```python
from build123d import *

# Parameters (mm, degrees)
SKETCH1_W           = 73
SKETCH1_H           = 7.175
BOSS_EXTRUDE1_DEPTH = 6
SKETCH15_W          = 4
SKETCH15_H          = 1
BOSS_EXTRUDE6_DEPTH = 1
BOSS_EXTRUDE7_START = -0.5
BOSS_EXTRUDE7_DEPTH = 7.175


with BuildPart() as part:
    # Sketch1 → Boss-Extrude1 (new body)
    with BuildSketch(Plane(origin=(0, 0, 0), x_dir=(1, 0, 0), z_dir=(0, 1, 0))):
        with Locations((0, -3.0875)):
            Rectangle(SKETCH1_W, SKETCH1_H)
    extrude(amount=BOSS_EXTRUDE1_DEPTH)

    # Sketch15 → Boss-Extrude6 (add)
    with BuildSketch(Plane(origin=(0, 6, 0), x_dir=(1, 0, 0), z_dir=(0, 1, 0))):
        with Locations((2.25, 0)):
            Rectangle(SKETCH15_W, SKETCH15_H)
        with Locations((6.75, 0)):
            Rectangle(SKETCH15_W, SKETCH15_H)
        with Locations((11.25, 0)):
            Rectangle(SKETCH15_W, SKETCH15_H)
        with Locations((15.75, 0)):
            Rectangle(SKETCH15_W, SKETCH15_H)
        with Locations((20.25, 0)):
            Rectangle(SKETCH15_W, SKETCH15_H)
        with Locations((24.75, 0)):
            Rectangle(SKETCH15_W, SKETCH15_H)
        with Locations((29.25, 0)):
            Rectangle(SKETCH15_W, SKETCH15_H)
        with Locations((33.75, 0)):
            Rectangle(SKETCH15_W, SKETCH15_H)
        with Locations((-33.75, 0)):
            Rectangle(SKETCH15_W, SKETCH15_H)
        with Locations((-29.25, 0)):
            Rectangle(SKETCH15_W, SKETCH15_H)
        with Locations((-24.75, 0)):
            Rectangle(SKETCH15_W, SKETCH15_H)
        with Locations((-20.25, 0)):
            Rectangle(SKETCH15_W, SKETCH15_H)
        with Locations((-15.75, 0)):
            Rectangle(SKETCH15_W, SKETCH15_H)
        with Locations((-11.25, 0)):
            Rectangle(SKETCH15_W, SKETCH15_H)
        with Locations((-6.75, 0)):
            Rectangle(SKETCH15_W, SKETCH15_H)
        with Locations((-2.25, 0)):
            Rectangle(SKETCH15_W, SKETCH15_H)
    extrude(amount=BOSS_EXTRUDE6_DEPTH)

    # Sketch16 → Boss-Extrude7 (add)
    with BuildSketch(Plane.XY.offset(BOSS_EXTRUDE7_START)):
        with BuildLine():
            Line((-2.54, -6), (-2.54, -9))
            Line((-2.54, -9), (-6, -9))
            Line((-6, -9), (-6, 0))
            Line((-6, 0), (6, 0))
            Line((6, 0), (6, -9))
            Line((6, -9), (2.54, -9))
            Line((2.54, -9), (2.54, -6))
            ThreePointArc((2.54, -6), (0, -3.46), (-2.54, -6))
        make_face()
    extrude(amount=BOSS_EXTRUDE7_DEPTH)


solid = part.part
```
Here's how the part is built. I have some questions about the finished solid (model axes, mm). A direction names the side the tool comes from. Give positions to 0.01 mm unless a question says otherwise; leave off trailing zeros. Loops run counter-clockwise (first coordinate to the right, second up) from the corner with the lowest first, then second, coordinate; pieces in that order, holes last. Notation, with made-up numbers: M 18,3.5 L 48,3.5 A15 ccw 48,21.5 Z; hole C 14.5,58.25 d6. An arc over 180 degrees is marked long. Put each result on its own line as item: value. Start each with the question number.
(1) Will these pins go through, and if not, where does the flat tip stop? pin 1 Ø0.5 at (y, z) = (6.5, 0) entering from -X; pin 2 Ø0.8 at (x, y) = (-11, 6.5) entering from +Z; pin 3 Ø4 at (x, z) = (11, 4) entering from +Y.
(2) I need wall thicknesses on line 1 along X through (y, z) = (-8, 3.75); line 2 along X through (y, z) = (-1, 3); line 3 along Y through (x, z) = (32.5, 0). Which ranges of each line are inside material? Lowest first, please. Write a range as [from, to].
(3) For faces 4 (the flat face through (-36.5, 3, 3)), 5 (the flat face through (2.54, -8, 3)), 6 (the flat face through (21, 0, 3)), 7 (the flat face through (-21, 0, 3)), 8 (the flat face through (4, -9, 3)), which set-ups out of +Z, -Z, +X, -X, +Y, -Y let a thin tool reach every point of the face, with its end or its side?
(4) If we mould it in two halves opening along X, with no side actions, what happens to faces 1 (the flat face through (-2.54, -7, 3)), 2 (the flat face through (-1, 2, -0.5)), 3 (the flat face through (6, -4, 3))? For each: +X half, -X half, draft (parallel to the pull), parting line (faces both ways), or undercut.
(5) I want a section at A-A on z = 1.75. Please give me the cut outline in (x, y), then the cut area to 3 significant figures.
(6) I want a section at B-B on x = 29.5. Please give me the cut outline in (y, z) (3 decimals).
Answer block:
1. pin 1: x = -35.75
1. pin 2: z = 0.5
1. pin 3: y = 6
2. line 1: [-6, -2.54], [2.54, 6]
2. line 2: [-6, 6]
2. line 3: [0, 7]
3. face 4: +Z, -Z, -X, +Y, -Y
3. face 5: +Z, -Z, -Y
3. face 6: +Z, -Z, +X, -Y
3. face 7: +Z, -Z, -X, -Y
3. face 8: +Z, -Z, +X, -X, -Y
4. face 1: undercut
4. face 2: draft
4. face 3: +X half
5. outline: M -36.5,0 L -6,0 L -6,-9 L -2.54,-9 L -2.54,-6 A2.54 cw 2.54,-6 L 2.54,-9 L 6,-9 L 6,0 L 36.5,0 L 36.5,6 L -36.5,6 Z
5. area: 521 mm^2
6. outline: M 0,-0.5 L 7,-0.5 L 7,0.5 L 6,0.5 L 6,6.675 L 0,6.675 Z
